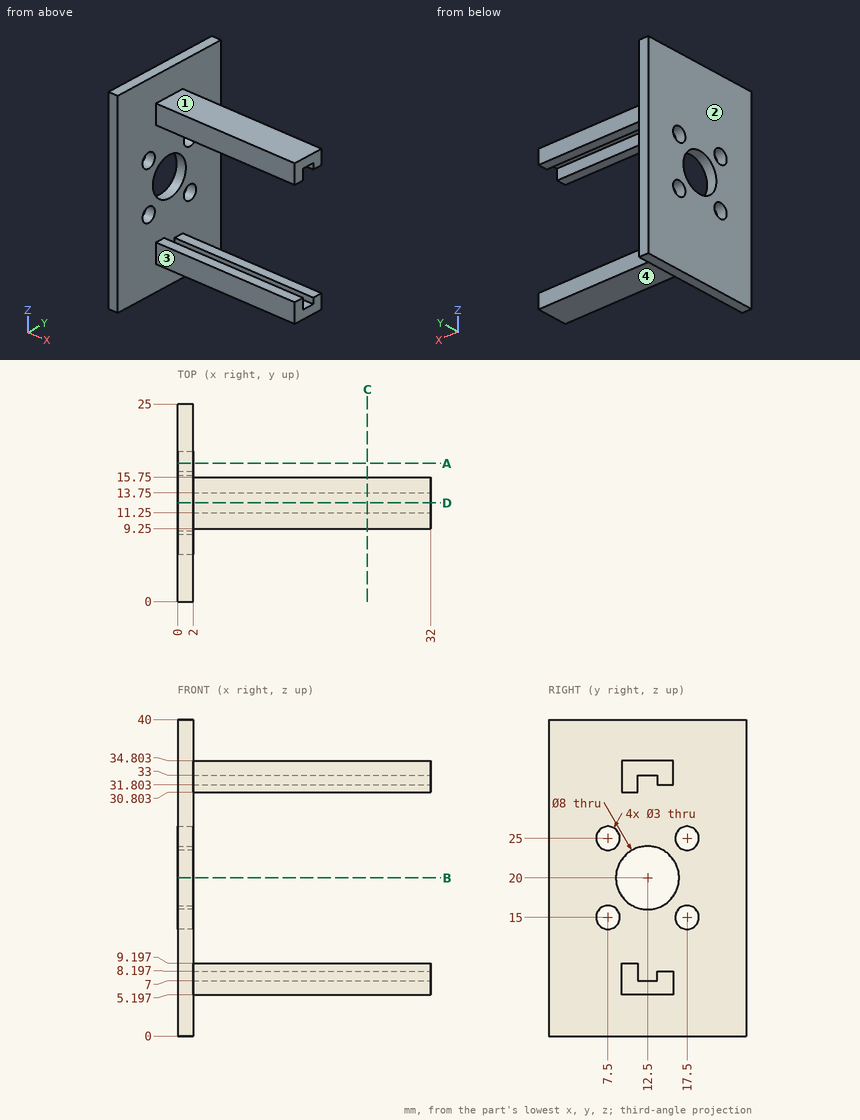
Input: dimensioned drawing with shaded views. Units: mm. Origin: part minimum x, y, z. A direction names the side the tool comes from. Coordinates: 2 decimals unless noted, no trailing zeros. Order: outer loops, then holes, each group sorted by start corner. A loop starts at its lowest first (then second) coordinate and runs counter-clockwise, first axis right, second up. Notation, with made-up numbers: M -12.5,7 L 17.5,7 A16 ccw 17.5,35 Z; hole C 34.25,-10 d9. An arc over 180 degrees is marked long. Answer as CSV lines item,"result".
Q1. First-contact query: P1, Ø2, axis at x = 25.5, z = 8, coming from the -Y side; P2, Ø0.9, axis at x = 21.5, z = 33.5, coming from the +Y side; P3, Ø2, axis at x = 18, y = 13, coming from the +Z side; P4, Ø2.5, axis at y = 7.5, z = 25, coming from the -X side. Flat tips, straight axial feed; report the tip coordinate or a pass-through.
Answers:
P1,"stops at y = 9.25"
P2,"stops at y = 15.75"
P3,"stops at z = 34.8"
P4,"passes through"
Q2. Section C-C on x = 24. Return the cut outline in (y, z), and give its area (3 significant figures).
Answers:
outline,"M 9.25,5.2 L 15.75,5.2 L 15.75,8.2 L 13.75,8.2 L 13.75,7 L 11.25,7 L 11.25,9.2 L 9.25,9.2 Z; M 9.25,30.8 L 11.25,30.8 L 11.25,33 L 13.75,33 L 13.75,31.8 L 15.75,31.8 L 15.75,34.8 L 9.25,34.8 Z"
area,"37.0 mm^2"
Q3. Line query: probe 1 along Y at (x, z) = (1, 25); probe 2 along Z at (x, y) = (21, 14.5); probe 3 along Z at (x, y) = (21.5, 13.5). Output: solid intervals per line, ascending. Write a range as [from, to].
Answers:
probe 1,"y = [0, 6], [9, 16], [19, 25]"
probe 2,"z = [5.2, 8.2], [31.8, 34.8]"
probe 3,"z = [5.2, 7], [33, 34.8]"
Q4. Section B-B on z = 20. Return the cut outline in (x, y).
Answers:
outline,"M 0,0 L 2,0 L 2,8.5 L 0,8.5 Z; M 0,16.5 L 2,16.5 L 2,25 L 0,25 Z"
Q5. Set-up query: the marked faces 1, 2, 3 and 4. Return all of +Z, -Z, +X, -X, +Y, -Y with unobstructed straight access to the full face (end or side cutting, diameter ignored); none if empty.
Answers:
face 1,"+Z, +X, +Y, -Y"
face 2,"+Z, -Z, -X, +Y, -Y"
face 3,"+Z, -Z, +X, -Y"
face 4,"-Z, +X, +Y, -Y"
Q6. Section D-D on y = 12.5. Return the cut outline in (x, z).
Answers:
outline,"M 0,0 L 2,0 L 2,5.2 L 32,5.2 L 32,7 L 2,7 L 2,16 L 0,16 Z; M 0,24 L 2,24 L 2,33 L 32,33 L 32,34.8 L 2,34.8 L 2,40 L 0,40 Z"
Q7. Section A-A on y = 17.5. Return the cut outline in (x, z).
Answers:
outline,"M 0,0 L 2,0 L 2,13.5 L 0,13.5 Z; M 0,16.5 L 2,16.5 L 2,23.5 L 0,23.5 Z; M 0,26.5 L 2,26.5 L 2,40 L 0,40 Z"
